```python
from build123d import *

# Parameters (mm, degrees)
SKETCH1_R           = 92.71
SKETCH1_R_2         = 53.975
BOSS_EXTRUDE1_DEPTH = 3.175
SKETCH2_R           = 92.71
SKETCH2_R_2         = 89.71
BOSS_EXTRUDE2_DEPTH = 266.7
SKETCH3_R           = 9.525
CUT_EXTRUDE1_DEPTH  = 270.875


with BuildPart() as part:
    # Sketch1 → Boss-Extrude1 (new body)
    with BuildSketch(Plane(origin=(0, 0, 0), x_dir=(1, 0, 0), z_dir=(0, 1, 0))):
        Circle(SKETCH1_R)
        Circle(SKETCH1_R_2, mode=Mode.SUBTRACT)
    extrude(amount=BOSS_EXTRUDE1_DEPTH)

    # Sketch2 → Boss-Extrude2 (add)
    with BuildSketch(Plane(origin=(0, 3.175, 0), x_dir=(1, 0, 0), z_dir=(0, 1, 0))):
        Circle(SKETCH2_R)
        Circle(SKETCH2_R_2, mode=Mode.SUBTRACT)
    extrude(amount=BOSS_EXTRUDE2_DEPTH)

    # Sketch3 → Cut-Extrude1 (cut, through all)
    with BuildSketch(Plane.XZ):
        with Locations((-80.264, 0)):
            Circle(SKETCH3_R)
        with Locations((80.264, 0)):
            Circle(SKETCH3_R)
    extrude(amount=-CUT_EXTRUDE1_DEPTH, mode=Mode.SUBTRACT)


solid = part.part
```
Input: part model. Units: mm. Frame: model coordinates. A direction names the side the tool comes from. Give positions to 0.01 mm unless a question says otherwise; leave off trailing zeros. Order: outer loops, then holes, each group sorted by start corner. A loop starts at its lowest first (then second) coordinate and runs counter-clockwise, first axis right, second up.
1. Cut plane B-B (z = 24). Return loops of the section in (x, y) (3 decimals), and give its area (3 significant figures).
Computed:
outline: (-89.55, 0) - (-48.346, 0) - (-48.346, 3.175) - (-86.44, 3.175) - (-86.44, 269.875) - (-89.55, 269.875) - close; (48.346, 0) - (89.55, 0) - (89.55, 269.875) - (86.44, 269.875) - (86.44, 3.175) - (48.346, 3.175) - close
area: 1,920 mm2
2. Draft query along X for faces 3 (the face through (-39.78, 1.57, -36.48)), 4 (the face through (40, 0, 40)), 5 (the face through (-1.95, 134.66, 89.69)), 6 (the face through (85.64, 133.05, 35.51)). Return one class per face: released by +X, released by -X, zero draft, split by the parting line, or undercut.
Computed:
face 3: undercut
face 4: zero draft
face 5: undercut
face 6: split by the parting line
3. Set-up query: faces 1 (the face through (89.74, 134.31, 0.97)), 2 (the face through (1.95, 134.66, -89.69)). Return all of +Z, -Z, +X, -X, +Y, -Y with unobstructed straight access to the full face (end or side cutting, diameter ignored); none if empty.
Computed:
face 1: +Y, -Y
face 2: +Y
4. Line query: probe 1 along Y at (x, z) = (-44, -34) (3 decimals); probe 2 along X at (y, z) = (114.5, 15); probe 3 along Z at (x, y) = (58, 27). Output: solid intervals per line, ascending.
Computed:
probe 1: y = 0 to 3.175
probe 2: x = -91.49 to -88.45, 88.45 to 91.49
probe 3: z = -72.33 to -68.44, 68.44 to 72.33
5. Cut plane D-D (z = -63). Return loops of the section in (x, y) (3 decimals).
Computed:
outline: (-68.016, 0) - (68.016, 0) - (68.016, 269.875) - (63.866, 269.875) - (63.866, 3.175) - (-63.866, 3.175) - (-63.866, 269.875) - (-68.016, 269.875) - close
6. Pin query (flat end, axial travel): pin 1 Ø4 at (x, y) = (9, 210) entering from +Z; pin 2 Ø3 at (y, z) = (78, 33.5) entering from +X; pin 3 Ø3 at (y, z) = (127.5, -45) entering from +X. Return the tip coordinate at first contact, or that it passes through.
Computed:
pin 1: stops at z = 92.45
pin 2: stops at x = 87.01
pin 3: stops at x = 81.87
7. Cut plane A-A (x = 0). Return loops of the section in (y, z) (3 decimals).
Computed:
outline: (0, -92.71) - (269.875, -92.71) - (269.875, -89.71) - (3.175, -89.71) - (3.175, -53.975) - (0, -53.975) - close; (0, 53.975) - (3.175, 53.975) - (3.175, 89.71) - (269.875, 89.71) - (269.875, 92.71) - (0, 92.71) - close
